Check sheet for the modelled part. Datum: model origin and axes. Units: mm. Round coordinates to 2 decimals unless told otherwise and drop trailing zeros. Order: outer loops, then holes, each group sorted by start corner. A loop starts at its lowest first (then second) coordinate and runs counter-clockwise, first axis right, second up.
Q1. Cross-section at C-C on y = 21.5. Record the cut outline in (x, z), then the cut area to 3 significant figures.
Q2. Depth check by flat-ended pin: P1, Ø5, axis at x = -5.5, z = 4, coming from the +Y side; P2, Ø12, axis at x = 11, y = 11.5, coming from the -Z side; P3, Ø10, axis at y = 8.5, z = 0.5, coming from the -X side; P4, Ø1.5, axis at x = -6.5, y = 21, coming from the -Z side. Enter the tip coordinate at first touch or a pass-through.
Q3. Cross-section at A-A on x = 0. Record the cut outline in (y, z).
Q4. Mould release check, pull along Z, two halves, no side actions. Record for faces 1 (the cylindrical face through (-14.274, 12.558, -3.17)), 2 (the flat face through (-11, 25.4, -2)), 3 (the cylindrical face through (-5.05, 12.842, -6.587)): +Z half, -Z half, draft (parallel to the pull), parting line (faces both ways), or undercut.
Q5. Scan lines: probe 1 along X at (y, z) = (18, 0); probe 2 along Z at (x, y) = (-1.75, 5.5); probe 3 along X at (y, z) = (13, -2.5). Record each from-to range of solid material in increasing order.
Q6. Cross-section at B-B on z = 0. Record the cut outline in (x, y).
from build123d import *

# Parameters (mm, degrees)
SKETCH1_R           = 14.622116372
BOSS_EXTRUDE2_DEPTH = 25.4
SKETCH2_R           = 8.3
CUT_EXTRUDE1_DEPTH  = 25.4
FILLET1_R           = 2.54


with BuildPart() as part:
    # Sketch1 → Boss-Extrude2 (new body)
    with BuildSketch(Plane(origin=(0, 0, 0), x_dir=(1, 0, 0), z_dir=(0, 1, 0))):
        with Locations(Location((0, 0, 0), (0, 0, 270))):
            Circle(SKETCH1_R)
    extrude(amount=BOSS_EXTRUDE2_DEPTH)

    # Sketch2 → Cut-Extrude1 (cut)
    with BuildSketch(Plane(origin=(0, 25.4, 0), x_dir=(1, 0, 0), z_dir=(0, 1, 0))):
        with Locations(Location((0, 0, 0), (0, 0, 270))):
            Circle(SKETCH2_R)
    extrude(amount=-CUT_EXTRUDE1_DEPTH, mode=Mode.SUBTRACT)

    # Fillet1
    fillet1_edges = [part.edges().sort_by_distance(p)[0] for p in [
        (0, 0, -14.622116372),
        (0, 25.4, -14.622116372),
        (0, 0, -8.3),
        (0, 25.4, -8.3),
    ]]
    fillet(fillet1_edges, radius=FILLET1_R)


solid = part.part
Results found:
1. outline: circle Ø29.24 at (0, 0); hole circle Ø16.6 at (0, 0)
1. area: 455 mm2
2. P1: stops at y = 24.88
2. P2: stops at z = -13.74
2. P3: stops at x = -14.62
2. P4: stops at z = -13.44
3. outline: (0, -12.08) arc R2.54 ccw to (2.54, -14.62) - (22.86, -14.62) arc R2.54 ccw to (25.4, -12.08) - (25.4, -10.84) arc R2.54 ccw to (22.86, -8.3) - (2.54, -8.3) arc R2.54 ccw to (0, -10.84) - close; (0, 10.84) arc R2.54 ccw to (2.54, 8.3) - (22.86, 8.3) arc R2.54 ccw to (25.4, 10.84) - (25.4, 12.08) arc R2.54 ccw to (22.86, 14.62) - (2.54, 14.62) arc R2.54 ccw to (0, 12.08) - close
4. face 1: parting line
4. face 2: draft
4. face 3: undercut
5. probe 1: x = -14.62 to -8.3, 8.3 to 14.62
5. probe 2: z = -14.52 to -8.11, 8.11 to 14.52
5. probe 3: x = -14.41 to -7.91, 7.91 to 14.41
6. outline: (-14.62, 2.54) arc R2.54 ccw to (-12.08, 0) - (-10.84, 0) arc R2.54 ccw to (-8.3, 2.54) - (-8.3, 22.86) arc R2.54 ccw to (-10.84, 25.4) - (-12.08, 25.4) arc R2.54 ccw to (-14.62, 22.86) - close; (8.3, 2.54) arc R2.54 ccw to (10.84, 0) - (12.08, 0) arc R2.54 ccw to (14.62, 2.54) - (14.62, 22.86) arc R2.54 ccw to (12.08, 25.4) - (10.84, 25.4) arc R2.54 ccw to (8.3, 22.86) - close
